from build123d import *

# Parameters (mm, degrees)
SKETCH1_W                      = 60
SKETCH1_H                      = 90
SKETCH1_R                      = 1.5
BOSS_EXTRUDE1_DEPTH            = 1
BOSS_EXTRUDE2_DEPTH            = 16.5
SKETCH3_W                      = 2
SKETCH3_H                      = 90
BOSS_EXTRUDE3_DEPTH            = 13.5
BOSS_EXTRUDE4_DEPTH            = 1
SKETCH5_W                      = 13.1
SKETCH5_H                      = 3
SKETCH5_W_2                    = 13.7
CUT_EXTRUDE1_DEPTH             = 16.5
SKETCH6_W                      = 15.9
SKETCH6_H                      = 3
CUT_EXTRUDE2_DEPTH             = 14.5
SKETCH7_R                      = 1.5
SKETCH7_W                      = 6.6
SKETCH7_H                      = 6.6
SKETCH7_H_2                    = 5.6
BOSS_EXTRUDE5_DEPTH            = 16.5
FILLET3_R                      = 3
CUT_EXTRUDE3_DEPTH             = 78.24797732
CUT_EXTRUDE3_DEPTH_BACK        = 2
SKETCH10_W                     = 2
SKETCH10_H                     = 15.2
CUT_EXTRUDE4_DEPTH             = 3.43
SKETCH11_W                     = 2
SKETCH11_H                     = 7.7
BOSS_EXTRUDE6_DEPTH            = 0.35
SKETCH13_W                     = 90
SKETCH13_H                     = 70
BOSS_EXTRUDE7_DEPTH            = 2
SKETCH14_W                     = 90
SKETCH14_H                     = 70
SKETCH14_W_2                   = 84
SKETCH14_H_2                   = 64
BOSS_EXTRUDE8_DEPTH            = 16.5
SKETCH15_W                     = 86
SKETCH15_H                     = 66
SKETCH15_W_2                   = 84
SKETCH15_H_2                   = 64
SKETCH15_W_3                   = 4
SKETCH15_H_3                   = 1
BOSS_EXTRUDE9_DEPTH            = 1
SKETCH16_W                     = 6
SKETCH16_H                     = 64
CUT_EXTRUDE6_DEPTH             = 1
CUT_EXTRUDE7_REACH             = 142.151
SKETCH17_R                     = 6
CUT_EXTRUDE7_DIRECTION_2_DEPTH = 141.150811628
BOSS_EXTRUDE10_DEPTH           = 16.5
CUT_EXTRUDE8_DEPTH             = 56
CUT_EXTRUDE8_DEPTH_BACK        = 19
SKETCH18_R                     = 1.5
SKETCH20_W                     = 6
SKETCH20_H                     = 50.8
CUT_EXTRUDE9_DEPTH             = 16.5
FILLET4_R                      = 0.5
FILLET5_R                      = 0.5
CUT_EXTRUDE10_DEPTH            = 4


with BuildPart() as part:
    # Sketch1 → Boss-Extrude1 (new, symmetric)
    with BuildSketch(Plane.XY):
        Rectangle(SKETCH1_W, SKETCH1_H)
        with Locations((-24.2, -18.8)):
            Circle(SKETCH1_R, mode=Mode.SUBTRACT)
        with Locations((-24.2, 39.2)):
            Circle(SKETCH1_R, mode=Mode.SUBTRACT)
        with Locations((24.8, 39.2)):
            Circle(SKETCH1_R, mode=Mode.SUBTRACT)
        with Locations((24.8, -18.8)):
            Circle(SKETCH1_R, mode=Mode.SUBTRACT)
    extrude(amount=BOSS_EXTRUDE1_DEPTH, both=True)

    # Sketch2 → Boss-Extrude2 (add)
    with BuildSketch(Plane.XY.offset(1)):
        Polygon((-27, 42), (28, 42), (28, 45), (-30, 45), (-30, -45), (28, -45), (28, -42), (-27, -42), align=None)
    extrude(amount=BOSS_EXTRUDE2_DEPTH)

    # Sketch3 → Boss-Extrude3 (add)
    with BuildSketch(Plane.XY.offset(1)):
        with Locations((29, 0)):
            Rectangle(SKETCH3_W, SKETCH3_H)
    extrude(amount=BOSS_EXTRUDE3_DEPTH)

    # Sketch4 → Boss-Extrude4 (add)
    with BuildSketch(Plane.XY.offset(17.5)):
        Polygon((28, -43), (-28, -43), (-28, 43), (28, 43), (28, 42), (-27, 42), (-27, -42), (28, -42), align=None)
    extrude(amount=BOSS_EXTRUDE4_DEPTH)

    # Sketch5 → Cut-Extrude1 (cut)
    with BuildSketch(Plane.XY.offset(18.5)):
        with Locations((-18.92, -43.5)):
            Rectangle(SKETCH5_W, SKETCH5_H)
        with Locations((-0.82, -43.5)):
            Rectangle(SKETCH5_W_2, SKETCH5_H)
    extrude(amount=-CUT_EXTRUDE1_DEPTH, mode=Mode.SUBTRACT)

    # Sketch6 → Cut-Extrude2 (cut)
    with BuildSketch(Plane.XY.offset(18.5)):
        with Locations((17.98, -43.5)):
            Rectangle(SKETCH6_W, SKETCH6_H)
    extrude(amount=-CUT_EXTRUDE2_DEPTH, mode=Mode.SUBTRACT)

    # Sketch7 → Boss-Extrude5 (add)
    # profile 1 of 4: a face of its own
    with BuildSketch(Plane.XY.offset(1)):
        with BuildLine():
            Line((-27, -15.9), (-23.3, -15.9))
            ThreePointArc((-23.3, -15.9), (-20.4, -18.8), (-23.3, -21.7))
            Line((-23.3, -21.7), (-27, -21.7))
            Line((-27, -21.7), (-27, -15.9))
        make_face()
        with Locations((-24.2, -18.8)):
            Circle(SKETCH7_R, mode=Mode.SUBTRACT)
    # profile 2 of 4: a face of its own
    with BuildSketch(Plane.XY.offset(1)):
        with Locations((-23.7, 38.7)):
            Rectangle(SKETCH7_W, SKETCH7_H)
        with Locations((-24.2, 39.2)):
            Circle(SKETCH7_R, mode=Mode.SUBTRACT)
    # profile 3 of 4: a face of its own
    with BuildSketch(Plane.XY.offset(1)):
        with BuildLine():
            Line((24.3, -21.7), (28, -21.7))
            Line((28, -21.7), (28, -15.9))
            Line((28, -15.9), (24.3, -15.9))
            ThreePointArc((24.3, -15.9), (21.4, -18.8), (24.3, -21.7))
        make_face()
        with Locations((24.8, -18.8)):
            Circle(SKETCH7_R, mode=Mode.SUBTRACT)
    # profile 4 of 4: a face of its own
    with BuildSketch(Plane.XY.offset(1)):
        with Locations((24.7, 39.2)):
            Rectangle(SKETCH7_W, SKETCH7_H_2)
        with Locations((24.8, 39.2)):
            Circle(SKETCH7_R, mode=Mode.SUBTRACT)
    extrude(amount=BOSS_EXTRUDE5_DEPTH)

    # Fillet3
    fillet3_edges = [part.edges().sort_by_distance(p)[0] for p in [
        (-20.4, 35.4, 9.25),
        (21.4, 36.4, 9.25),
    ]]
    fillet(fillet3_edges, radius=FILLET3_R)

    # Sketch9 → Cut-Extrude3 (cut, two sides: drawn at the far end of the back side and taken through both)
    with BuildSketch(Plane(origin=(30, 0, 0), x_dir=(0, 0, -1), z_dir=(1, 0, 0)).offset(-CUT_EXTRUDE3_DEPTH_BACK)):
        with BuildLine():
            Line((-146.271990211, -13.88), (-14.5, -13.88))
            ThreePointArc((-14.5, -13.88), (-11.3, -10.68), (-14.5, -7.48))
            Line((-14.5, -7.48), (-146.271990211, -7.48))
            Line((-146.271990211, -7.48), (-409.815970634, -7.48))
            Line((-409.815970634, -7.48), (-409.815970634, -13.88))
            Line((-409.815970634, -13.88), (-146.271990211, -13.88))
        make_face()
    extrude(amount=CUT_EXTRUDE3_DEPTH + CUT_EXTRUDE3_DEPTH_BACK, mode=Mode.SUBTRACT)

    # Sketch10 → Cut-Extrude4 (cut)
    with BuildSketch(Plane.XY.offset(14.5)):
        with Locations((29, 10.98)):
            Rectangle(SKETCH10_W, SKETCH10_H)
    extrude(amount=-CUT_EXTRUDE4_DEPTH, mode=Mode.SUBTRACT)

    # Sketch11 → Boss-Extrude6 (add)
    with BuildSketch(Plane.XY.offset(14.5)):
        with Locations((29, 32.32)):
            Rectangle(SKETCH11_W, SKETCH11_H)
    extrude(amount=BOSS_EXTRUDE6_DEPTH)

    # Sketch13 → Boss-Extrude7 (add)
    with BuildSketch(Plane(origin=(0, 0, -1), x_dir=(-1, 0, 0), z_dir=(0, 0, -1))):
        with Locations((75, 10)):
            Rectangle(SKETCH13_W, SKETCH13_H)
    extrude(amount=-BOSS_EXTRUDE7_DEPTH)

    # Sketch14 → Boss-Extrude8 (add)
    with BuildSketch(Plane.XY.offset(1)):
        with Locations((-75, 10)):
            Rectangle(SKETCH14_W, SKETCH14_H)
        with Locations((-75, 10)):
            Rectangle(SKETCH14_W_2, SKETCH14_H_2, mode=Mode.SUBTRACT)
    extrude(amount=BOSS_EXTRUDE8_DEPTH)

    # Sketch15 → Boss-Extrude9 (add)
    # profile 1 of 3: a face of its own
    with BuildSketch(Plane.XY.offset(17.5)):
        with Locations((-75, 10)):
            Rectangle(SKETCH15_W, SKETCH15_H)
        with Locations((-75, 10)):
            Rectangle(SKETCH15_W_2, SKETCH15_H_2, mode=Mode.SUBTRACT)
    # profile 2 of 3: a face of its own
    with BuildSketch(Plane.XY.offset(17.5)):
        with Locations((-30, -22.5)):
            Rectangle(SKETCH15_W_3, SKETCH15_H_3)
    # profile 3 of 3: a face of its own
    with BuildSketch(Plane.XY.offset(17.5)):
        with Locations((-30, 42.5)):
            Rectangle(SKETCH15_W_3, SKETCH15_H_3)
    extrude(amount=BOSS_EXTRUDE9_DEPTH)

    # Sketch16 → Cut-Extrude6 (cut)
    with BuildSketch(Plane.XY.offset(18.5)):
        with Locations((-30, 10)):
            Rectangle(SKETCH16_W, SKETCH16_H)
    extrude(amount=-CUT_EXTRUDE6_DEPTH, mode=Mode.SUBTRACT)

    # Sketch17 → Cut-Extrude7 (cut, up to next)
    with BuildSketch(Plane.XZ.offset(25), mode=Mode.PRIVATE) as cut_extrude7_sk1:
        with Locations(Location((-45, 8.25, 0), (0, 0, 90))):
            Circle(SKETCH17_R)
    cut_extrude7_tool1 = extrude(cut_extrude7_sk1.sketch, amount=-CUT_EXTRUDE7_REACH, mode=Mode.PRIVATE) & part.part
    # Sketch17 → Cut-Extrude7 (cut, up to next)
    with BuildSketch(Plane.XZ.offset(25), mode=Mode.PRIVATE) as cut_extrude7_sk2:
        with Locations(Location((-65, 8.25, 0), (0, 0, 90))):
            Circle(SKETCH17_R)
    cut_extrude7_tool2 = extrude(cut_extrude7_sk2.sketch, amount=-CUT_EXTRUDE7_REACH, mode=Mode.PRIVATE) & part.part
    # Sketch17 → Cut-Extrude7 (cut, up to next)
    with BuildSketch(Plane.XZ.offset(25), mode=Mode.PRIVATE) as cut_extrude7_sk3:
        with Locations(Location((-85, 8.25, 0), (0, 0, 90))):
            Circle(SKETCH17_R)
    cut_extrude7_tool3 = extrude(cut_extrude7_sk3.sketch, amount=-CUT_EXTRUDE7_REACH, mode=Mode.PRIVATE) & part.part
    # Sketch17 → Cut-Extrude7 (cut, up to next)
    with BuildSketch(Plane.XZ.offset(25), mode=Mode.PRIVATE) as cut_extrude7_sk4:
        with Locations(Location((-105, 8.25, 0), (0, 0, 90))):
            Circle(SKETCH17_R)
    cut_extrude7_tool4 = extrude(cut_extrude7_sk4.sketch, amount=-CUT_EXTRUDE7_REACH, mode=Mode.PRIVATE) & part.part
    add(cut_extrude7_tool1.solids().sort_by_distance((-45, -25, 8.25))[0], mode=Mode.SUBTRACT)
    add(cut_extrude7_tool2.solids().sort_by_distance((-65, -25, 8.25))[0], mode=Mode.SUBTRACT)
    add(cut_extrude7_tool3.solids().sort_by_distance((-85, -25, 8.25))[0], mode=Mode.SUBTRACT)
    add(cut_extrude7_tool4.solids().sort_by_distance((-105, -25, 8.25))[0], mode=Mode.SUBTRACT)

    # Sketch17 → Cut-Extrude7 direction 2 (cut)
    with BuildSketch(Plane.XZ.offset(25)):
        with Locations(Location((-45, 8.25, 0), (0, 0, 90))):
            Circle(SKETCH17_R)
        with Locations(Location((-65, 8.25, 0), (0, 0, 90))):
            Circle(SKETCH17_R)
        with Locations(Location((-85, 8.25, 0), (0, 0, 90))):
            Circle(SKETCH17_R)
        with Locations(Location((-105, 8.25, 0), (0, 0, 90))):
            Circle(SKETCH17_R)
    extrude(amount=CUT_EXTRUDE7_DIRECTION_2_DEPTH, mode=Mode.SUBTRACT)

    # Sketch19 → Boss-Extrude10 (add)
    with BuildSketch(Plane.XY.offset(1)):
        with BuildLine():
            Line((-117, -15.400002114), (-113.400002114, -15.400002114))
            ThreePointArc((-113.400002114, -15.400002114), (-111.27868177, -16.27868177), (-110.400002114, -18.400002114))
            Line((-110.400002114, -18.400002114), (-110.400002114, -22))
            Line((-110.400002114, -22), (-117, -22))
            Line((-117, -22), (-117, -15.400002114))
        make_face()
        with BuildLine():
            Line((-40.6, -22), (-40.6, -18.4))
            ThreePointArc((-40.6, -18.4), (-39.721320344, -16.278679656), (-37.6, -15.4))
            Line((-37.6, -15.4), (-33, -15.4))
            Line((-33, -15.4), (-33, -22))
            Line((-33, -22), (-40.6, -22))
        make_face()
        with BuildLine():
            Line((-39.6, 42), (-39.6, 38.4))
            ThreePointArc((-39.6, 38.4), (-38.721320344, 36.278679656), (-36.6, 35.4))
            Line((-36.6, 35.4), (-33, 35.4))
            Line((-33, 35.4), (-33, 42))
            Line((-33, 42), (-39.6, 42))
        make_face()
        with BuildLine():
            Line((-110.4, 42), (-110.4, 38.4))
            ThreePointArc((-110.4, 38.4), (-111.278679656, 36.278679656), (-113.4, 35.4))
            Line((-113.4, 35.4), (-117, 35.4))
            Line((-117, 35.4), (-117, 42))
            Line((-117, 42), (-110.4, 42))
        make_face()
    extrude(amount=BOSS_EXTRUDE10_DEPTH)

    # Sketch18 → Cut-Extrude8 (cut, two sides: drawn at the far end of the back side and taken through both)
    with BuildSketch(Plane.XY.offset(1).offset(-CUT_EXTRUDE8_DEPTH_BACK)):
        with Locations((-114.2, 39.2)):
            Circle(SKETCH18_R)
        with Locations((-35.8, 39.2)):
            Circle(SKETCH18_R)
        with Locations((-35.8, -19.2)):
            Circle(SKETCH18_R)
        with Locations((-114.2, -19.2)):
            Circle(SKETCH18_R)
    extrude(amount=CUT_EXTRUDE8_DEPTH + CUT_EXTRUDE8_DEPTH_BACK, mode=Mode.SUBTRACT)

    # Sketch20 → Cut-Extrude9 (cut)
    with BuildSketch(Plane.XY.offset(17.5)):
        with Locations((-30, 10)):
            Rectangle(SKETCH20_W, SKETCH20_H)
    extrude(amount=-CUT_EXTRUDE9_DEPTH, mode=Mode.SUBTRACT)

    # Fillet4
    fillet4_edges = [part.edges().sort_by_distance(p)[0] for p in [
        (-27, -15.9, 9.25),
    ]]
    fillet(fillet4_edges, radius=FILLET4_R - 0.0001)  # a hair under: the kernel refuses the full size

    # Fillet5
    fillet5_edges = [part.edges().sort_by_distance(p)[0] for p in [
        (-27, -15.4, 9.25),
    ]]
    fillet(fillet5_edges, radius=FILLET5_R)

    # Sketch21 → Cut-Extrude10 (cut)
    with BuildSketch(Plane(origin=(0, 45, 0), x_dir=(1, 0, 0), z_dir=(0, 1, 0))):
        with BuildLine():
            Line((-110, -17.5), (-110, -18.5))
            Line((-110, -18.5), (-100, -18.5))
            Line((-100, -18.5), (-100, -17.5))
            ThreePointArc((-100, -17.5), (-105, -12.5), (-110, -17.5))
        make_face()
    extrude(amount=-CUT_EXTRUDE10_DEPTH, mode=Mode.SUBTRACT)


solid = part.part
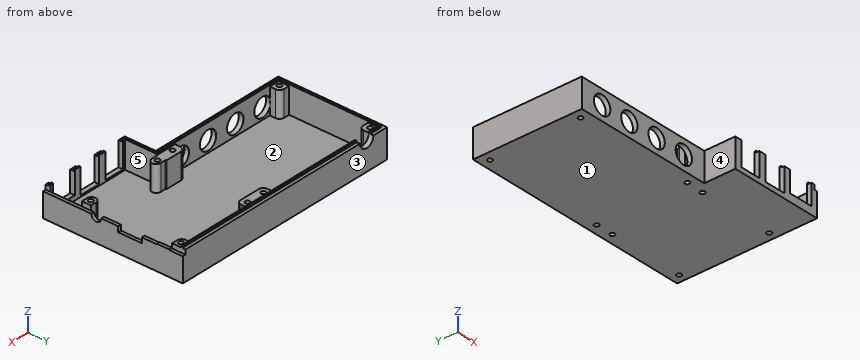
Work out the finished part from the listing and answer in its coordinate system (mm). Face numbers are marked on the shaded views. A direction names the side the tool comes from. Give positions to 0.01 mm unless a question says otherwise; leave off trailing zeros. Loops run counter-clockwise (first coordinate to the right, second up) from the corner with the lowest first, then second, coordinate; pieces in that order, holes last. Notation, with made-up numbers: (56, -30) -> (109, -30) arc R32 cw to (109, 9) -> close; hole circle Ø7 at (64, 42). An arc over 180 degrees is marked (long way). Use a Markdown table: item, result. Add a question column.
1. Determine the mould class of the marked faces 3, 4 and 5 for opening direction Y: released by +Y, released by -Y, zero draft, split by the parting line, or undercut.
2. Find the intervals of material crossed by probe 1 along Y at (x, z) = (-24.2, 6.25); probe 2 along Y at (x, z) = (-29.5, 11); probe 3 along Z at (x, y) = (-105, -24), in increasing order.
3. Section A-A on x = -45 is taken. Determine the outline of the cut face in (y, z).
4. Section B-B on y = 10.5 is taken. Determine the outline of the cut face in (x, z), and give its area (3 significant figures).
5. For the marked faces 1 and 2, determine the directions among +Z, -Z, +X, -X, +Y, -Y from which every point of the face is accessible in a straight line to the end or side of a thin tool.
6. Section C-C on z = 7.5 is taken. State how many separate pieces and enclosed holes the cut face has, and give its area (3 significant figures).
7. Flat-ended cylindrical pins translate along their axes: pin 1 Ø0.5 at (y, z) = (-35.5, 18) entering from -X; pin 2 Ø0.6 at (x, y) = (-59, 44) entering from +Z; pin 3 Ø1.1 at (x, z) = (-89.5, 18) entering from -Y. Find the tip coordinate at first contact, or state that the pin passes through.
8. Section D-D on x = -105 is taken. Determine the outline of the cut face in (y, z), and give its area (3 significant figures).
Results below:
| question | item | result |
|---|---|---|
| 1 | face 3 | released by +Y |
| 1 | face 4 | zero draft |
| 1 | face 5 | undercut |
| 2 | probe 1 | y = -21.7 to -20.3, -17.3 to -15.9, 35.4 to 37.7, 40.7 to 45 |
| 2 | probe 2 | y = -45 to -15.4, 35.4 to 45 |
| 2 | probe 3 | z = -1 to 2.25, 14.25 to 17.5 |
| 3 | outline | (-25, -1) -> (45, -1) -> (45, 17.5) -> (43, 17.5) -> (43, 18.5) -> (42, 18.5) -> (42, 1) -> (-22, 1) -> (-22, 2.25) -> (-25, 2.25) -> close; (-25, 14.25) -> (-22, 14.25) -> (-22, 18.5) -> (-23, 18.5) -> (-23, 17.5) -> (-25, 17.5) -> close |
| 4 | outline | (-120, -1) -> (30, -1) -> (30, 11.07) -> (28, 11.07) -> (28, 1) -> (-117, 1) -> (-117, 18.5) -> (-118, 18.5) -> (-118, 17.5) -> (-120, 17.5) -> close |
| 4 | area | 371 mm^2 |
| 5 | face 1 | -Z, +X, -X, +Y, -Y |
| 5 | face 2 | +Z |
| 6 | separate pieces | 7 |
| 6 | enclosed holes | 8 |
| 6 | area | 1,390 mm^2 |
| 7 | pin 1 | stops at x = -28 |
| 7 | pin 2 | stops at z = 17.5 |
| 7 | pin 3 | stops at y = -25 |
| 8 | outline | (-25, -1) -> (45, -1) -> (45, 12.5) -> (42, 12.5) -> (42, 1) -> (-22, 1) -> (-22, 2.25) -> (-25, 2.25) -> close; (-25, 14.25) -> (-22, 14.25) -> (-22, 18.5) -> (-23, 18.5) -> (-23, 17.5) -> (-25, 17.5) -> close |
| 8 | area | 189 mm^2 |
